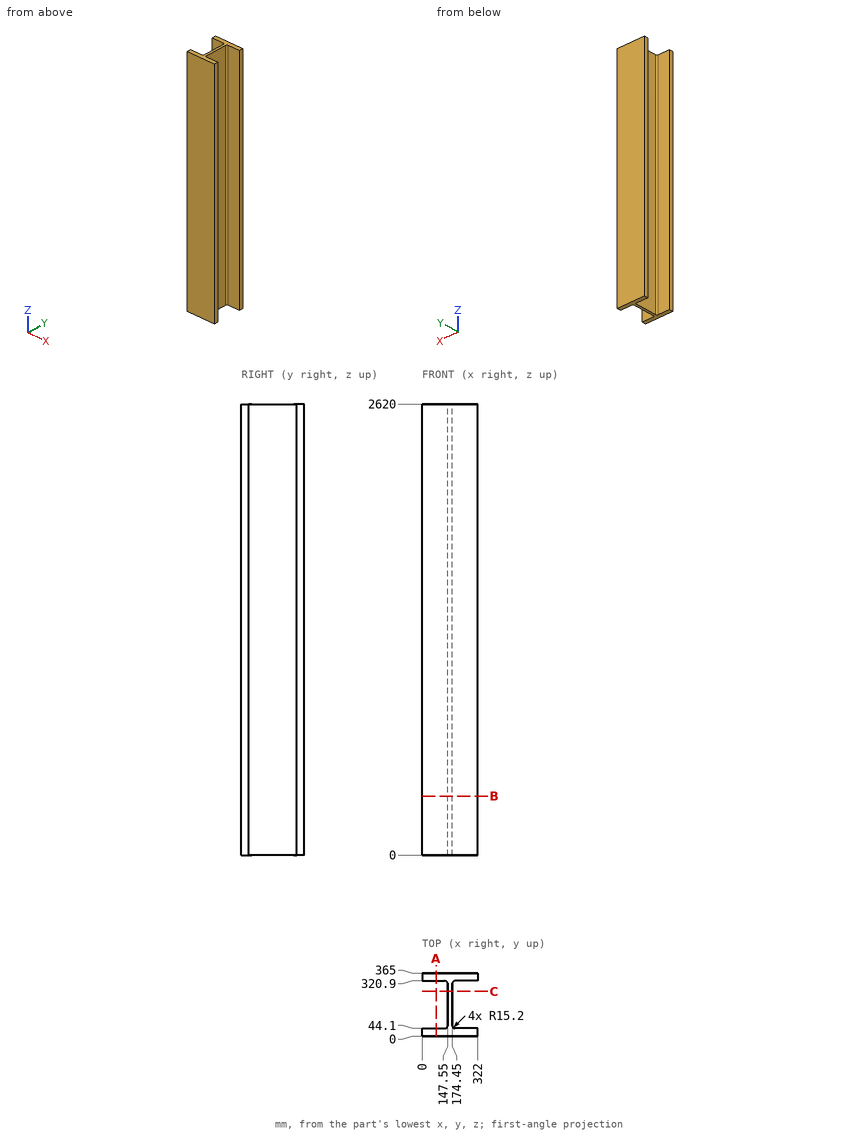
Input: dimensioned drawing with shaded views. Units: mm. Origin: part minimum x, y, z. Give positions to 0.01 mm unless a question says otherwise; leave off trailing zeros. Write each loop counter-clockwise with the first axis right and the second up, starting at its lowest first coordinate (ties: lowest second). Pieces come first, ordered by that corner, then holes. Notation, with made-up numbers: (84, 61) -> (139, 61) arc R16 ccw to (139, 72) -> close; hole circle Ø8 at (37.5, 88). An arc over 180 degrees is marked (long way). Return JSON: item names as keys, results as strings. Group by question number.
1. Pin query (flat end, axial travel): pin 1 Ø12 at (y, z) = (239, 1101.5) entering from +X; pin 2 Ø10 at (x, z) = (209.5, 2112.5) entering from -Y. Return the tip coordinate at first contact, or that it passes through.
2. Material intervals for line 1 (Y direction, x = 255, z = 2122); line 2 (X direction, y = 252, z = 538); line 3 (X direction, y = 309.5, z = 2278), sorted ascending. Write a range as from..to.
3. Section C-C, the plane y = 258.5. Output: boundary loops of the cut face in (x, z), then the cut area to 3 significant figures.
4. Section B-B, the plane z = 343. Output: boundary loops of the cut face in (x, y).
5. Section A-A, the plane x = 81.5. Output: boundary loops of the cut face in (y, z), then the cut area to 3 significant figures.
Determined:
{
 "1": {"pin 1": "stops at x = 174.45", "pin 2": "stops at y = 0"},
 "2": {"line 1": "y = 0..44.1, 320.9..365", "line 2": "x = 147.55..174.45", "line 3": "x = 147.07..174.93"},
 "3": {"outline": "(147.55, 0) -> (174.45, 0) -> (174.45, 2620) -> (147.55, 2620) -> close", "area": "70,500 mm2"},
 "4": {"outline": "(0, 0) -> (322, 0) -> (322, 44.1) -> (189.65, 44.1) arc R15.2 cw to (174.45, 59.3) -> (174.45, 305.7) arc R15.2 cw to (189.65, 320.9) -> (322, 320.9) -> (322, 365) -> (0, 365) -> (0, 320.9) -> (132.35, 320.9) arc R15.2 cw to (147.55, 305.7) -> (147.55, 59.3) arc R15.2 cw to (132.35, 44.1) -> (0, 44.1) -> close"},
 "5": {"outline": "(0, 0) -> (44.1, 0) -> (44.1, 2620) -> (0, 2620) -> close; (320.9, 0) -> (365, 0) -> (365, 2620) -> (320.9, 2620) -> close", "area": "231,000 mm2"}
}
